Input: dimensioned drawing with shaded views. Units: mm. Origin: part minimum x, y, z. Round coordinates to 2 decimals unless told otherwise and drop trailing zeros. Order: outer loops, then holes, each group sorted by start corner. A loop starts at its lowest first (then second) coordinate and runs counter-clockwise, first axis right, second up. Notation, with made-up numbers: M -31.75,-37.75 L -1.75,-37.75 A25 ccw -1.75,-24.75 Z; hole C 81,-36.75 d8. An arc over 180 degrees is marked long. One line per question, with ' | ' between items.
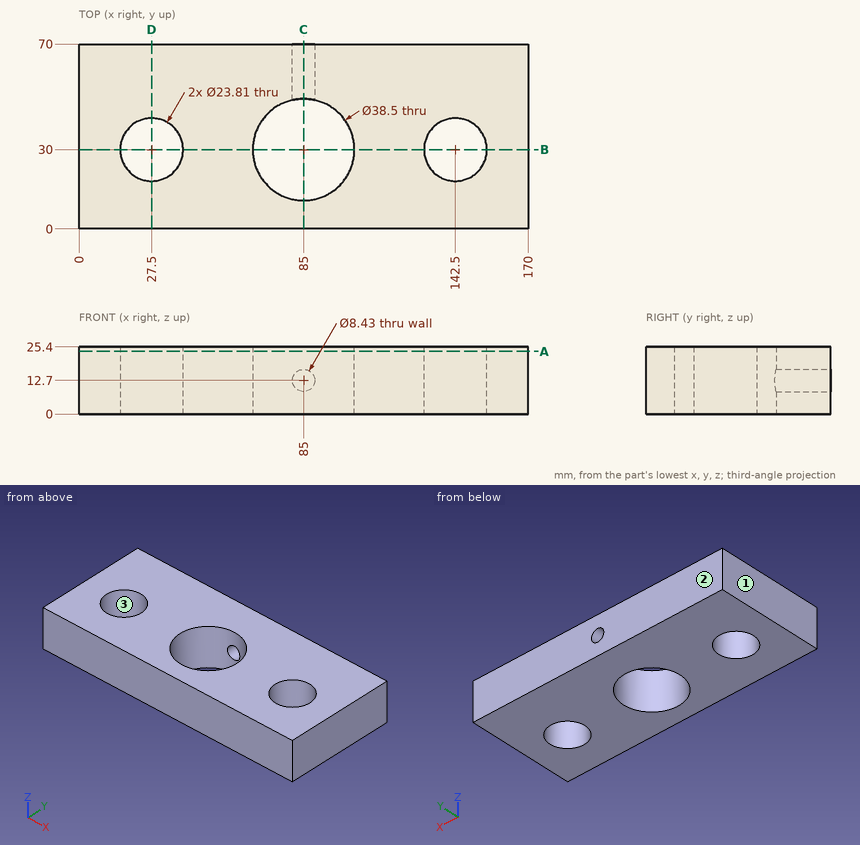
Item 1: First-contact query: pin 1 (21.5 mm diameter, centred on x = 142.5, y = 30, fed in from +Z); pin 2 (7.5 mm diameter, centred on x = 85, z = 12.7, fed in from +Y); pin 3 (3 mm diameter, centred on x = 72.5, z = 9, fed in from -Y). Flat tips, straight axial feed; report the tip coordinate or a pass-through.
Report:
pin 1: through | pin 2: y = 11.12 | pin 3: y = 0
Item 2: Mould query, pull axis Y, two halves, no side actions, for the marked faces 1, 2 and 3. Classes: +Y half, -Y half, draft (parallel to the pull), parting line (faces both ways), or undercut.
Report:
face 1: draft | face 2: +Y half | face 3: undercut
Item 3: Section query C-C, the plane x = 85. Return loops of the section in (y, z) (3 decimals).
Report:
outline: M 0,0 L 10.75,0 L 10.75,25.4 L 0,25.4 Z; M 49.25,0 L 70,0 L 70,8.485 L 49.25,8.485 Z; M 49.25,16.915 L 70,16.915 L 70,25.4 L 49.25,25.4 Z
Item 4: Section query D-D, the plane x = 27.5. Return loops of the section in (y, z) (3 decimals), plus the area to 3 significant figures.
Report:
outline: M 0,0 L 18.095,0 L 18.095,25.4 L 0,25.4 Z; M 41.905,0 L 70,0 L 70,25.4 L 41.905,25.4 Z | area: 1,170 mm²
Item 5: Section query A-A, the plane z = 23.75. Return loops of the section in (x, y) (3 decimals).
Report:
outline: M 0,0 L 170,0 L 170,70 L 0,70 Z; hole C 27.5,30 d23.81; hole C 85,30 d38.5; hole C 142.5,30 d23.81
Item 6: Section query B-B, the plane y = 30. Return loops of the section in (x, z) (3 decimals), plus the area to 3 significant figures.
Report:
outline: M 0,0 L 15.595,0 L 15.595,25.4 L 0,25.4 Z; M 39.405,0 L 65.75,0 L 65.75,25.4 L 39.405,25.4 Z; M 104.25,0 L 130.595,0 L 130.595,25.4 L 104.25,25.4 Z; M 154.405,0 L 170,0 L 170,25.4 L 154.405,25.4 Z | area: 2,130 mm²
Item 7: Line query: line 1 along Y through (x, z) = (142.5, 11.25) (3 decimals); line 2 along X through (y, z) = (26, 19.5); line 3 along Z through (x, y) = (85, 60.5) (3 decimals). Output: solid intervals per line, ascending. Write a range as from..to.
Report:
line 1: 0..18.095, 41.905..70 | line 2: 0..16.29, 38.71..66.17, 103.83..131.29, 153.71..170 | line 3: 0..8.485, 16.915..25.4
